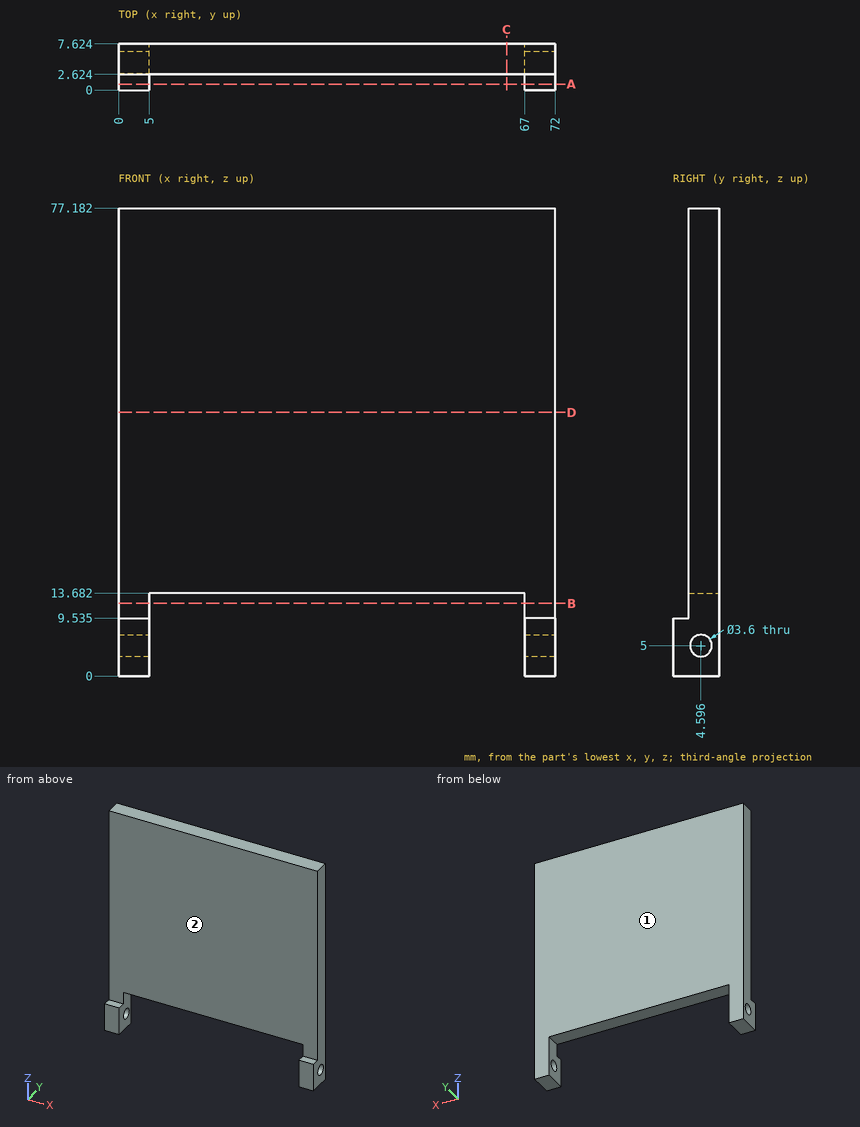
Print and shaded views of the part. All mm, measured from the part's lowest x, y and z. A direction names the side the tool comes from. Coordinates: 2 decimals unless noted, no trailing zeros. Write each loop counter-clockwise with the first axis right and the second up, starting at its lowest first coordinate (ties: lowest second). Pieces come first, ordered by that corner, then holes. Notation, with made-up numbers: (63, -34) -> (97, -34) arc R6 ccw to (97, -28) -> close; hole circle Ø3 at (-34.75, 50). An arc over 180 degrees is marked (long way). Use CSV: the item, a comma, the result in double quotes. Start each with the question number.
Q1. Drill centre lines: probe 1 along Y at (x, z) = (34.5, 22); probe 2 along Z at (x, y) = (51, 7.25); probe 3 along Z at (x, y) = (67.5, 3.25) (1 decimal). Where is each one in solid material? Low to high.
Q2. Cut at B-B, the plane z = 12. List the corners of the cut face in (x, y), then the cut area to 3 significant figures.
Q3. Cut at A-A, the plane y = 1. List the corners of the cut face in (x, z) (1 decimal).
Q4. 3-axis set-ups, long thin cutter, end or side, ignore diameter. For the marked faces 1 and 2: which of +Z, -Z, +X, -X, +Y, -Y reach the whole face in a straight line?
Q5. Flat gauge pins, fed straight in: pin 1 Ø2 at (x, y) = (3.5, 1) entering from +Z (1 decimal); pin 2 Ø2 at (y, z) = (1.5, 61) entering from -X; pin 3 Ø2.5 at (x, y) = (36, 4.5) entering from -Z. Where does each tip first touch, or does it go through?
Q6. Cut at C-C, the plane x = 64. List the corners of the cut face in (y, z).
Q7. Cut at D-D, the plane z = 43.5. List the corners of the cut face in (x, y), then the cut area to 3 significant figures.
Checked values:
1,probe 1,"y = 2.62 to 7.62"
1,probe 2,"z = 13.68 to 77.18"
1,probe 3,"z = 0 to 3.8, 6.2 to 77.2"
2,outline,"(0, 2.62) -> (5, 2.62) -> (5, 7.62) -> (0, 7.62) -> close; (67, 2.62) -> (72, 2.62) -> (72, 7.62) -> (67, 7.62) -> close"
2,area,"50.0 mm²"
3,outline,"(0, 0) -> (5, 0) -> (5, 9.5) -> (0, 9.5) -> close; (67, 0) -> (72, 0) -> (72, 9.5) -> (67, 9.5) -> close"
4,face 1,"+Z, -Z, +X, -X, +Y"
4,face 2,"+Z, +X, -X, -Y"
5,pin 1,"stops at z = 9.5"
5,pin 2,"passes through"
5,pin 3,"stops at z = 13.68"
6,outline,"(2.62, 13.68) -> (7.62, 13.68) -> (7.62, 77.18) -> (2.62, 77.18) -> close"
7,outline,"(0, 2.62) -> (72, 2.62) -> (72, 7.62) -> (0, 7.62) -> close"
7,area,"360 mm²"
